from build123d import *

# Parameters (mm, degrees)
F1_DEPTH = 25.4


with BuildPart() as f1:
    # F0 (on Front) → F1 (new body)
    with BuildSketch(Plane.XZ):
        with BuildLine():
            Line((-17.578895, 7.366), (-17.578895, 0))
            Line((-17.578895, 0), (-17.578895, -7.366))
            ThreePointArc((-17.578895, -7.366), (-16.834947, -9.162051), (-15.038895, -9.906))
            Line((-15.038895, -9.906), (2.741105, -9.906))
            ThreePointArc((2.741105, -9.906), (3.63913, -9.534026), (4.011105, -8.636))
            Line((4.011105, -8.636), (4.011105, -5.221252))
            ThreePointArc((4.011105, -5.221252), (4.2608, -4.427238), (5.020116, -4.086291))
            Line((5.020116, -4.086291), (5.020116, -8.128))
            Line((5.020116, -8.128), (11.631105, -8.128))
            Line((11.631105, -8.128), (18.242093, -8.128))
            Line((18.242093, -8.128), (18.242093, -4.086291))
            ThreePointArc((18.242093, -4.086291), (19.001409, -4.427238), (19.251105, -5.221252))
            Line((19.251105, -5.221252), (19.251105, -8.636))
            ThreePointArc((19.251105, -8.636), (19.623079, -9.534026), (20.521105, -9.906))
            Line((20.521105, -9.906), (38.301105, -9.906))
            ThreePointArc((38.301105, -9.906), (40.097156, -9.162051), (40.841105, -7.366))
            Line((40.841105, -7.366), (40.841105, 0))
            Line((40.841105, 0), (40.841105, 7.366))
            ThreePointArc((40.841105, 7.366), (40.097156, 9.162051), (38.301105, 9.906))
            Line((38.301105, 9.906), (20.521105, 9.906))
            ThreePointArc((20.521105, 9.906), (19.623079, 9.534026), (19.251105, 8.636))
            Line((19.251105, 8.636), (19.251105, 5.221252))
            ThreePointArc((19.251105, 5.221252), (19.001409, 4.427238), (18.242093, 4.086291))
            Line((18.242093, 4.086291), (18.242093, 8.128))
            Line((18.242093, 8.128), (11.631105, 8.128))
            Line((11.631105, 8.128), (5.020116, 8.128))
            Line((5.020116, 8.128), (5.020116, 4.086291))
            ThreePointArc((5.020116, 4.086291), (4.2608, 4.427238), (4.011105, 5.221252))
            Line((4.011105, 5.221252), (4.011105, 8.636))
            ThreePointArc((4.011105, 8.636), (3.63913, 9.534026), (2.741105, 9.906))
            Line((2.741105, 9.906), (-15.038895, 9.906))
            ThreePointArc((-15.038895, 9.906), (-16.834947, 9.162051), (-17.578895, 7.366))
        make_face()
    extrude(amount=F1_DEPTH)


solid = f1.part
Source: CAD feature listing. Evaluate the final solid. Frame: model axes, mm. A direction names the side the tool comes from. Round coordinates to 2 decimals unless told otherwise and drop trailing zeros. Loops run counter-clockwise (first coordinate to the right, second up) from the corner with the lowest first, then second, coordinate; pieces in that order, holes last.
Q1. Ray query, line 1 (X direction, y = -18.5, z = -6); line 2 (X direction, y = -9, z = -4.25); line 3 (Z direction, x = 8.5, y = -17.25). Return the intervals inside material, ascending.
Q2. Access query for faces 1 (the face through (40.841, -13, 0)), 2 (the face through (19.251, -13, 7)), 3 (the face through (5.02, -13, -6)). Directions: +Z, -Z, +X, -X, +Y, -Y. A direction counts if a zero-diameter tool reaches every point of the face in a straight line with its end or side. Return the directions, or none.
Q3. Section A-A, the plane y = -21.25. Return loops of the section in (x, z).
Q4. Section B-B, the plane x = 14. Return loops of the section in (y, z), plus the area to 3 significant figures.
Q5. Mould query, pull axis X, two halves, no side actions, for faces 4 (the face through (-17.579, -13, 0)), 5 (the face through (4.011, -13, 7)), 6 (the face through (11, 0, 0)), 7 (the face through (3.629, -12.522, -9.544)). Classes: pulls with the +X half, pulls with the -X half, needs draft (parallel to the pull), parting line crosses it, or undercut.
Q6. First-contact query: P1, Ø4, axis at x = 13.5, y = -13, coming from the +Z side; P2, Ø10.5, axis at x = 10.5, y = -12, coming from the -Z side; P3, Ø1, axis at y = -19, z = 8, coming from the +X side. Flat tips, straight axial feed; report the tip coordinate or a pass-through.
Solutions:
1. line 1: x = -17.58 to 4.01, 5.02 to 18.24, 19.25 to 40.84
1. line 2: x = -17.58 to 4.47, 5.02 to 18.24, 18.8 to 40.84
1. line 3: z = -8.13 to 8.13
2. face 1: +Z, -Z, +X, +Y, -Y
2. face 2: +Z, +Y, -Y
2. face 3: -Z, +Y, -Y
3. outline: (-17.58, -7.37) arc R2.54 ccw to (-15.04, -9.91) - (2.74, -9.91) arc R1.27 ccw to (4.01, -8.64) - (4.01, -5.22) arc R1.02 cw to (5.02, -4.09) - (5.02, -8.13) - (18.24, -8.13) - (18.24, -4.09) arc R1.02 cw to (19.25, -5.22) - (19.25, -8.64) arc R1.27 ccw to (20.52, -9.91) - (38.3, -9.91) arc R2.54 ccw to (40.84, -7.37) - (40.84, 7.37) arc R2.54 ccw to (38.3, 9.91) - (20.52, 9.91) arc R1.27 ccw to (19.25, 8.64) - (19.25, 5.22) arc R1.02 cw to (18.24, 4.09) - (18.24, 8.13) - (5.02, 8.13) - (5.02, 4.09) arc R1.02 cw to (4.01, 5.22) - (4.01, 8.64) arc R1.27 ccw to (2.74, 9.91) - (-15.04, 9.91) arc R2.54 ccw to (-17.58, 7.37) - close
4. outline: (-25.4, -8.13) - (0, -8.13) - (0, 8.13) - (-25.4, 8.13) - close
4. area: 413 mm2
5. face 4: pulls with the -X half
5. face 5: undercut
5. face 6: needs draft
5. face 7: undercut
6. P1: stops at z = 8.13
6. P2: stops at z = -8.13
6. P3: stops at x = 40.84
